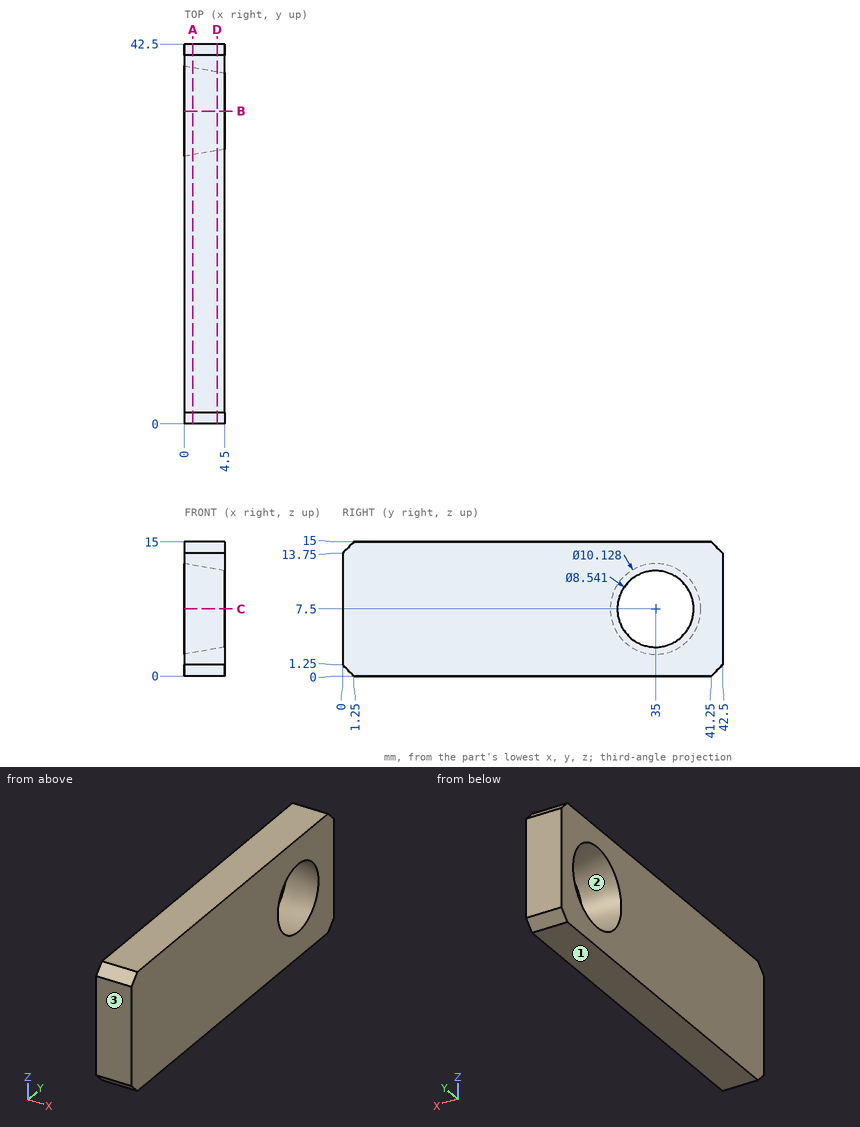
Verification items for this drawing (mm, ordinates from the low corner). Give positions to 0.01 mm unless a question says otherwise; leave off trailing zeros. Loops run counter-clockwise (first coordinate to the right, second up) from the corner with the lowest first, then second, coordinate; pieces in that order, holes last. Notation, with made-up numbers: M 78.5,-33.5 L 105.5,-33.5 A8 ccw 105.5,-23.5 Z; hole C 61,-28 d3. An arc over 180 degrees is marked long. Answer as a JSON object with one key per item and string values. Group by question number.
Item 1: Sectioned sample at A-A on x = 0.95. Record the boundary of the cut face in (y, z).
Item 2: Mould release check, pull along Z, two halves, no side actions. Record for the marked faces 1, 2 and 3: pulls with the +Z half, pulls with the -Z half, needs draft (parallel to the pull), parting line crosses it, or undercut.
Item 3: Sectioned sample at C-C on z = 7.5. Record the boundary of the cut face in (x, y), plus the area to 3 significant figures.
Item 4: Gauge pin test, flat end, axial feed: pin 1 (5 mm diameter, centred on y = 36, z = 2, fed in from -X). Record the tip position at first contact, or that the pin passes through.
Item 5: Sectioned sample at D-D on x = 3.65. Record the boundary of the cut face in (y, z), plus the area to 3 significant figures.
Item 6: Material ranges on L1, parallel to Y at x = 0.75, z = 7.75 (1 decimal); L2, parallel to Z at x = 1.8, y = 34; L3, parallel to Y at x = 2.75, z = 10.5, recorded low to high.
Item 7: Sectioned sample at B-B on y = 35. Record the boundary of the cut face in (x, z), plus the area to 3 significant figures.
Findings below:
{
 "1": {"outline": "M 0,1.25 L 1.25,0 L 41.25,0 L 42.5,1.25 L 42.5,13.75 L 41.25,15 L 1.25,15 L 0,13.75 Z; hole C 35,7.5 d9.79"},
 "2": {"face 1": "pulls with the -Z half", "face 2": "undercut", "face 3": "needs draft"},
 "3": {"outline": "M 0,0 L 4.5,0 L 4.5,30.73 L 0,29.94 Z; M 0,40.06 L 4.5,39.27 L 4.5,42.5 L 0,42.5 Z", "area": "149 mm2"},
 "4": {"pin 1": "x = 0"},
 "5": {"outline": "M 0,1.25 L 1.25,0 L 41.25,0 L 42.5,1.25 L 42.5,13.75 L 41.25,15 L 1.25,15 L 0,13.75 Z; hole C 35,7.5 d8.84", "area": "573 mm2"},
 "6": {"L1": "0 to 30.1, 39.9 to 42.5", "L2": "0 to 2.86, 12.14 to 15", "L3": "0 to 31.54, 38.46 to 42.5"},
 "7": {"outline": "M 0,0 L 4.5,0 L 4.5,3.23 L 0,2.44 Z; M 0,12.56 L 4.5,11.77 L 4.5,15 L 0,15 Z", "area": "25.5 mm2"}
}
